from build123d import *
from build123d.topology import SkipClean

# Parameters (mm, degrees)
ESQUISSE1_R          = 5
ESQUISSE1_R_2        = 1.55
BOSS_EXTRU_1_DEPTH   = 9.8
BOSS_EXTRUDE7_DEPTH  = 9.8
CUT_EXTRUDE3_DEPTH   = 2
SKETCH14_R           = 1.55
BOSS_EXTRUDE11_DEPTH = 1.5
BOSS_EXTRUDE12_DEPTH = 3
BOSS_EXTRUDE17_START = -1
BOSS_EXTRUDE17_DEPTH = 3
FILLET3_R            = 1
FILLET5_R            = 1


with BuildPart() as part:
    # Esquisse1 → Boss.-Extru.1 (new body)
    with BuildSketch(Plane.XY):
        Circle(ESQUISSE1_R)
        Circle(ESQUISSE1_R_2, mode=Mode.SUBTRACT)
    extrude(amount=BOSS_EXTRU_1_DEPTH)

    # Sketch8 → Boss-Extrude7 (add)
    with BuildSketch(Plane(origin=(0, 0, 0), x_dir=(-1, 0, 0), z_dir=(0, 0, -1))):
        with BuildLine():
            Line((0, 5), (-14.046192928, 5))
            ThreePointArc((-14.046192928, 5), (-19.046192928, 0), (-14.046192928, -5))
            Line((-14.046192928, -5), (0, -5))
            ThreePointArc((0, -5), (-5, 0), (0, 5))
        make_face()
    extrude(amount=-BOSS_EXTRUDE7_DEPTH)

    # Sketch12 → Cut-Extrude3 (cut)
    with SkipClean():  # the faces are left unmerged after this step: merging them gives an invalid solid
        with BuildSketch(Plane(origin=(0, 0, 0), x_dir=(-1, 0, 0), z_dir=(0, 0, -1))):
            with BuildLine():
                Line((-14.046192928, 5), (-7.023096464, 5))
                Line((-7.023096464, 5), (0, 5))
                ThreePointArc((0, 5), (-5, 0), (0, -5))
                Line((0, -5), (-7.023096464, -5))
                Line((-7.023096464, -5), (-14.046192928, -5))
                ThreePointArc((-14.046192928, -5), (-19.046192928, 0), (-14.046192928, 5))
            make_face()
        cut_extrude3 = extrude(amount=-CUT_EXTRUDE3_DEPTH, mode=Mode.SUBTRACT)

    # Mirror3: Cut-Extrude3 across plane
    with SkipClean():  # the faces are left unmerged after this step: merging them gives an invalid solid
        add(cut_extrude3.mirror(Plane.XY.offset(4.9)), mode=Mode.SUBTRACT)

    # Sketch14 → Boss-Extrude11 (add, symmetric)
    with SkipClean():  # the faces are left unmerged after this step: merging them gives an invalid solid
        with BuildSketch(Plane(origin=(0, 0, 0), x_dir=(1, 0, 0), z_dir=(0, 1, 0))):
            with BuildLine():
                Line((10.546192928, -2), (17.546192928, -2))
                Line((17.546192928, -2), (17.546192928, 0.5))
                ThreePointArc((17.546192928, 0.5), (14.046192928, 4), (10.546192928, 0.5))
                Line((10.546192928, 0.5), (10.546192928, -2))
            make_face()
            with Locations(Location((14.046192928, 0.5, 0), (0, 0, 180))):
                Circle(SKETCH14_R, mode=Mode.SUBTRACT)
        boss_extrude11 = extrude(amount=BOSS_EXTRUDE11_DEPTH, both=True)

    # Mirror4: Boss-Extrude11 across plane
    with SkipClean():  # the faces are left unmerged after this step: merging them gives an invalid solid
        add(boss_extrude11.mirror(Plane.XY.offset(4.9)))

    # Sketch15 → Boss-Extrude12 (add)
    with SkipClean():  # the faces are left unmerged after this step: merging them gives an invalid solid
        with BuildSketch(Plane(origin=(0, 1.5, 0), x_dir=(1, 0, 0), z_dir=(0, 1, 0))):
            with BuildLine():
                Line((10.546192928, 0.5), (10.546192928, 6.476059904))
                Line((10.546192928, 6.476059904), (17.546192928, 6.476059904))
                Line((17.546192928, 6.476059904), (17.546192928, 0.5))
                ThreePointArc((17.546192928, 0.5), (14.046192928, 4), (10.546192928, 0.5))
            make_face()
        extrude(amount=-BOSS_EXTRUDE12_DEPTH)

    # Sketch23 → Boss-Extrude17 (add)
    with SkipClean():  # the faces are left unmerged after this step: merging them gives an invalid solid
        with BuildSketch(Plane(origin=(0, 0, -6.476059904), x_dir=(-1, 0, 0), z_dir=(0, 0, -1)).offset(BOSS_EXTRUDE17_START)):
            Polygon((-17.546192928, 1.5), (-11.796192928, 2.565699508), (-11.796192928, 1.5), align=None)
        extrude(amount=-BOSS_EXTRUDE17_DEPTH)

    # Fillet3
    fillet3_edges = [part.edges().sort_by_distance(p)[0] for p in [
        (10.546192928, -1.5, 9.05),
        (17.546192928, -1.5, 9.05),
        (14.046192928, -1.5, 13.8),
        (10.546192928, 1.5, 9.05),
        (17.546192928, 1.5, 9.05),
        (14.046192928, 1.5, 13.8),
    ]]
    fillet(fillet3_edges, radius=FILLET3_R)

    # Fillet5
    fillet5_edges = [part.edges().sort_by_distance(p)[0] for p in [
        (14.046192928, -1.5, -6.476059904),
        (14.046192928, 1.5, -6.476059904),
        (17.546192928, 0, -6.476059904),
        (10.546192928, 0, -6.476059904),
        (10.546192928, 1.5, -2.238029952),
        (10.546192928, -1.5, -2.238029952),
        (17.546192928, -1.5, -2.238029952),
    ]]
    fillet(fillet5_edges, radius=FILLET5_R - 0.0001)  # a hair under: the kernel refuses the full size


solid = part.part
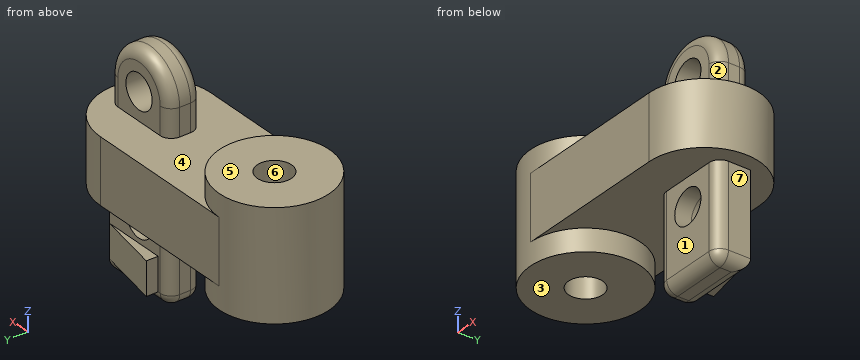
Could you check a few things on this model? Use its own coordinates, in mm. Face numbers are marked on the shaded views. A direction names the side the tool comes from. Give positions to 0.01 mm unless a question says otherwise; leave off trailing zeros. Write each loop counter-clockwise with the first axis right and the second up, starting at its lowest first coordinate (ties: lowest second). Pieces come first, ordered by that corner, then holes. Notation, with made-up numbers: (-24.5, -20.75) - (-8.5, -20.75) arc R20 ccw to (-8.5, -3.75) - close; hole circle Ø11 at (4.25, 46). An arc over 180 degrees is marked (long way). Use CSV: the item, a comma, the result in double quotes. Start each with the question number.
Item 1: I'm going to push flat-ended pins straight in: pin 1 (2.5 mm diameter, centred on x = 14, z = -3, fed in from -Y); pin 2 (5 mm diameter, centred on x = 2.5, y = -1, fed in from -Z); pin 3 (0.8 mm diameter, centred on y = 0, z = -1.5, fed in from -X). Where does each tip first touch, or does it pass through?
Item 2: If I drill on line 1 along Z through (x, y) = (14, -0.25); line 2 along Z through (x, y) = (14.75, 1); line 3 along Z through (x, y) = (14.25, -3.25), over which ranges is the centre line in solid material (lowest first)?
Item 3: I want a section at D-D, the plane y = -3.5. Please give me the cut outline in (x, z).
Item 4: I want a section at C-C, the plane z = 4.5. Please give me the cut outline in (x, y).
Item 5: If we mould it in two halves opening along X, with no side actions, what happens to the marked faces 4, 5, 6 and 7? For each: pulls with the +X half, pulls with the -X half, needs draft (parallel to the pull), parting line crosses it, or undercut.
Item 6: I want a section at A-A, the plane z = -0.5. Please give me the cut outline in (x, y), then the cut area to 3 significant figures.
Item 7: For the marked faces 1, 2 and 3, which set-ups out of +Z, -Z, +X, -X, +Y, -Y let a thin tool reach every point of the face, with its end or its side?
Item 8: I want a section at B-B, the plane x = -0.5. Please give me the cut outline in (y, z).
Findings:
1,pin 1,"stops at y = -1.5"
1,pin 2,"stops at z = 0"
1,pin 3,"stops at x = 10.55"
2,line 1,"z = -6.48 to -2.05, 1.05 to 8.75, 11.85 to 13.8"
2,line 2,"z = -6.34 to -1.88, 0.88 to 8.92, 11.68 to 13.59"
2,line 3,"z = 2 to 7.8"
3,outline,"(-3.57, 0) - (3.57, 0) - (3.57, 2) - (17.62, 2) - (17.62, 7.8) - (3.57, 7.8) - (3.57, 9.8) - (-3.57, 9.8) - close"
4,outline,"(0, -5) - (14.05, -5) arc R5 ccw to (14.05, 5) - (0, 5) arc R5 ccw to start; hole circle Ø3.1 at (0, 0)"
5,face 4,"undercut"
5,face 5,"needs draft"
5,face 6,"undercut"
5,face 7,"pulls with the +X half"
6,outline,"(10.55, -0.5) arc R1 ccw to (11.55, -1.5) - (12.5, -1.5) - (12.5, 1.5) - (11.55, 1.5) arc R1 ccw to (10.55, 0.5) - close; (15.6, -1.5) - (16.55, -1.5) arc R1 ccw to (17.55, -0.5) - (17.55, 1.5) - (15.6, 1.5) - close"
6,area,"11.1 mm2"
7,face 1,"-Z, +X, -Y"
7,face 2,"+Z, +X, -Y"
7,face 3,"-Z, -X, +Y, -Y"
8,outline,"(-4.97, 0) - (-1.47, 0) - (-1.47, 9.8) - (-4.97, 9.8) - close; (1.47, 0) - (4.97, 0) - (4.97, 9.8) - (1.47, 9.8) - close"
